The listing builds one solid part. Answer for the finished solid, in the listing's coordinates (mm). A direction names the side the tool comes from. Give positions to 0.01 mm unless a question says otherwise; leave off trailing zeros. Order: outer loops, then holes, each group sorted by start corner. A loop starts at its lowest first (then second) coordinate and runs counter-clockwise, first axis right, second up. Notation, with made-up numbers: (47.5, 82.5) -> (105.5, 82.5) arc R33 ccw to (105.5, 118.5) -> close; hole circle Ø2 at (63, -17.75). An arc over 180 degrees is marked (long way). Answer as a JSON object with one key per item and string values. Group by question number.
```python
from build123d import *

# Parameters (mm, degrees)
CYLINDER004_R     = 36.5
CYLINDER004_DEPTH = 4
CYLINDER005_R     = 38
CYLINDER005_DEPTH = 4
CYLINDER003_R     = 36.5
CYLINDER003_DEPTH = 4
CYLINDER002_R     = 38
CYLINDER002_DEPTH = 4
CYLINDER001_R     = 1.5
CYLINDER001_DEPTH = 40
CYLINDER_R        = 35
CYLINDER_DEPTH    = 35
PAD_DEPTH         = 1
SKETCH001_R       = 3
HOLE_DEPTH        = 25
PAD001_DEPTH      = 18
FILLET_1_R        = 1
FILLET_2_R        = 0.9
FILLET001_R       = 1
FILLET002_R       = 0.3


with BuildPart() as cylinder004:
    # Cylinder004 → Cylinder004 (new body)
    with BuildSketch(Plane(origin=(0, 0, -45), x_dir=(1, 0, 0), z_dir=(0, -1, 0))):
        Circle(CYLINDER004_R)
    extrude(amount=CYLINDER004_DEPTH)


with BuildPart() as cut003:
    # Cylinder005 → Cylinder005 (new body)
    with BuildSketch(Plane(origin=(0, 0, -45), x_dir=(1, 0, 0), z_dir=(0, -1, 0))):
        Circle(CYLINDER005_R)
    extrude(amount=CYLINDER005_DEPTH)

    # Cut003: cut Cylinder004
    add(cylinder004.part, mode=Mode.SUBTRACT)


with BuildPart() as cut003_1:
    # Cut003 placement: moved
    add(cut003.part.moved(Location((0, -12, 0))))


with BuildPart() as cylinder003:
    # Cylinder003 → Cylinder003 (new body)
    with BuildSketch(Plane(origin=(0, 0, -45), x_dir=(1, 0, 0), z_dir=(0, -1, 0))):
        Circle(CYLINDER003_R)
    extrude(amount=CYLINDER003_DEPTH)


with BuildPart() as fusion:
    # Cylinder002 → Cylinder002 (new body)
    with BuildSketch(Plane(origin=(0, 0, -45), x_dir=(1, 0, 0), z_dir=(0, -1, 0))):
        Circle(CYLINDER002_R)
    extrude(amount=CYLINDER002_DEPTH)

    # Cut002: cut Cylinder003
    add(cylinder003.part, mode=Mode.SUBTRACT)


with BuildPart() as fusion_1:
    # Cut002 placement: moved
    add(fusion.part.moved(Location((0, 6, 0))))

    # Fusion: union Cut003
    add(cut003_1.part)


with BuildPart() as cylinder001:
    # Cylinder001 → Cylinder001 (new body)
    with BuildSketch(Plane(origin=(-20, -15.75, -9.5), x_dir=(0, 0, -1), z_dir=(1, 0, 0))):
        Circle(CYLINDER001_R)
    extrude(amount=CYLINDER001_DEPTH)


with BuildPart() as cylinder:
    # Cylinder → Cylinder (new body)
    with BuildSketch(Plane(origin=(0, 12, -45), x_dir=(1, 0, 0), z_dir=(0, -1, 0))):
        Circle(CYLINDER_R)
    extrude(amount=CYLINDER_DEPTH)


with BuildPart() as fillet002:
    # Sketch → Pad (new body)
    with BuildSketch(Plane.XY):
        with BuildLine():
            ThreePointArc((-16, 10.5), (-18.474874, 9.474874), (-19.5, 7))
            Line((-19.5, 7), (-19.5, -17))
            ThreePointArc((-19.5, -17), (-18.474874, -19.474874), (-16, -20.5))
            Line((-16, -20.5), (15.999994, -20.5))
            ThreePointArc((15.999994, -20.5), (18.474872, -19.474876), (19.5, -17))
            Line((19.5, -17), (19.5, 7))
            ThreePointArc((19.5, 7), (18.474874, 9.474874), (16, 10.5))
            Line((16, 10.5), (-16, 10.5))
        make_face()
    extrude(amount=PAD_DEPTH)

    # Sketch001 (on Face9 of Pad) → Hole (cut)
    with BuildSketch(Plane(origin=(0, 0, 0), x_dir=(1, 0, 0), z_dir=(0, 0, -1))):
        Circle(SKETCH001_R)
    extrude(amount=-HOLE_DEPTH, mode=Mode.SUBTRACT)

    # Sketch002 (on Face4 of Hole) → Pad001 (join)
    with BuildSketch(Plane(origin=(0, 0, 0), x_dir=(1, 0, 0), z_dir=(0, 0, -1))):
        with BuildLine():
            Line((-16, 20.5), (15.999994, 20.5))
            ThreePointArc((19.5, 17), (18.474872, 19.474876), (15.999994, 20.5))
            Line((19.5, 17), (19.5, -7))
            ThreePointArc((16, -10.5), (18.474874, -9.474874), (19.5, -7))
            Line((16, -10.5), (-16, -10.5))
            ThreePointArc((-19.5, -7), (-18.474874, -9.474874), (-16, -10.5))
            Line((-19.5, -7), (-19.5, 17))
            ThreePointArc((-16, 20.5), (-18.474874, 19.474874), (-19.5, 17))
        make_face()
        with BuildLine():
            ThreePointArc((-18.5, -7), (-17.767767, -8.767767), (-16, -9.5))
            Line((16, -9.5), (-16, -9.5))
            ThreePointArc((16, -9.5), (17.767767, -8.767767), (18.5, -7))
            Line((18.5, 17), (18.5, -7))
            ThreePointArc((18.5, 17), (17.767767, 18.767767), (16, 19.5))
            Line((-15.993973, 19.5), (16, 19.5))
            ThreePointArc((-15.993973, 19.5), (-17.767772, 18.767772), (-18.5, 16.993973))
            Line((-18.5, -7), (-18.5, 16.993973))
        make_face(mode=Mode.SUBTRACT)
    extrude(amount=PAD001_DEPTH)

    # Cut: cut Cylinder
    add(cylinder.part, mode=Mode.SUBTRACT)

    # Cut001: cut Cylinder001
    add(cylinder001.part, mode=Mode.SUBTRACT)

    # Fillet 1
    fillet_1_edges = [fillet002.edges().sort_by_distance(p)[0] for p in [
        (0.003014, -19.5, 0),
    ]]
    fillet(fillet_1_edges, radius=FILLET_1_R)

    # Fillet 2
    fillet_2_edges = [fillet002.edges().sort_by_distance(p)[0] for p in [
        (19.5, -5, 1),
    ]]
    fillet(fillet_2_edges, radius=FILLET_2_R)

    # Cut004: cut Fusion
    add(fusion_1.part, mode=Mode.SUBTRACT)

    # Fillet001
    fillet001_edges = [fillet002.edges().sort_by_distance(p)[0] for p in [
        (-19.5, 4, -14.145503),
        (-19.5, -14, -14.145503),
        (19.5, -14, -14.145503),
        (19.5, 4, -14.145503),
    ]]
    fillet(fillet001_edges, radius=FILLET001_R)

    # Fillet002
    fillet002_edges = [fillet002.edges().sort_by_distance(p)[0] for p in [
        (-18.5, 4, -13.535735),
        (-18.5, -14, -13.535735),
        (18.5, -14, -13.535735),
        (18.5, 4, -13.535735),
    ]]
    fillet(fillet002_edges, radius=FILLET002_R)


solid = fillet002.part
```
(1) A cutting plane is placed at A-A (y = 3.5). Determine the outline of the cut face in (x, z), and give its area (3 significant figures).
(2) Flat-ended cylindrical pins translate along their axes: pin 1 Ø5 at (x, y) = (-2, -11) entering from -Z; pin 2 Ø0.5 at (x, z) = (19, -13.5) entering from -Y; pin 3 Ø0.5 at (x, z) = (19, -13.5) entering from +Y. Find the tip coordinate at first contact, or state that the pin passes through.
(3) A cutting plane is placed at C-C (y = 0). Determine the outline of the cut face in (x, z).
(4) A cutting plane is placed at D-D (z = -9.5). Determine the outline of the cut face in (x, y).
(5) Which of the six approach directions +Z, -Z, +X, -X, +Y, -Y give full straight-line access (tool end or side, diameter ignored) to faces 5 (the cylindrical face through (18.215, -4.832, -0.301)), 6 (the cylindrical face through (19.009, 4.028, -12.096)), 7 (the cylindrical face through (19, -15.7, -8))?
(6) For a pull along Z with two mould halves and no side action, classify faces 1 (the cylindrical face through (-0.22, 10.24, 0.73)), 2 (the cylindrical face through (-3, -0.1, 0.5)), 3 (the cylindrical face through (-19.376, 4.028, -14.218)), 4 (the cylindrical face through (0.227, -19.215, -0.301)) as +Z half, -Z half, draft (parallel to the pull), parting line (faces both ways), or undercut.
(7) Find the intervals of material crossed by line 1 along X through (y, z) = (3.5, -5.25); line 2 along Y through (x, z) = (14, -9); line 3 along Z through (x, y) = (14, 8), in increasing order. Write a range as [from, to].
(8) A cutting plane is placed at B-B (x = 0). Determine the outline of the cut face in (y, z), and give its area (3 significant figures).
Check sheet entries:
{
 "1": {"outline": "(-19.5, -15.94) arc R35 cw to (-18.5, -15.29) -> (-18.5, -14.06) arc R0.3 ccw to (-18.96, -13.81) arc R36.5 ccw to (-19.02, -13.85) arc R1 ccw to (-19.5, -14.7) -> close; (-19.5, -12.38) arc R38 cw to (-18.5, -11.81) -> (-18.5, -1) arc R1 cw to (-17.5, 0) -> (17.5, 0) arc R1 cw to (18.5, -1) -> (18.5, -11.81) arc R38 cw to (19.5, -12.38) -> (19.5, 0.1) arc R0.9 ccw to (18.6, 1) -> (-18.6, 1) arc R0.9 ccw to (-19.5, 0.1) -> close; (18.5, -15.29) arc R35 cw to (19.5, -15.94) -> (19.5, -14.7) arc R1 ccw to (19.02, -13.85) arc R36.5 ccw to (18.96, -13.81) arc R0.3 ccw to (18.5, -14.06) -> close", "area": "66.6 mm2"},
 "2": {"pin 1": "stops at z = 0", "pin 2": "stops at y = -19.17", "pin 3": "stops at y = 9.17"},
 "3": {"outline": "(-19.5, -15.94) arc R35 cw to (-18.5, -15.29) -> (-18.5, -1) arc R1 cw to (-17.5, 0) -> (-3, 0) -> (-3, 1) -> (-18.6, 1) arc R0.9 ccw to (-19.5, 0.1) -> close; (3, 0) -> (17.5, 0) arc R1 cw to (18.5, -1) -> (18.5, -15.29) arc R35 cw to (19.5, -15.94) -> (19.5, 0.1) arc R0.9 ccw to (18.6, 1) -> (3, 1) -> close"},
 "4": {"outline": "(-19.5, -14.25) -> (-18.5, -14.25) -> (-18.5, 7) arc R2.5 cw to (-16, 9.5) -> (16, 9.5) arc R2.5 cw to (18.5, 7) -> (18.5, -14.25) -> (19.5, -14.25) -> (19.5, 7) arc R3.5 ccw to (16, 10.5) -> (-16, 10.5) arc R3.5 ccw to (-19.5, 7) -> close; (-19.49, -17.25) arc R3.5 ccw to (-16, -20.5) -> (16, -20.5) arc R3.5 ccw to (19.49, -17.25) -> (18.49, -17.25) arc R2.5 cw to (16, -19.5) -> (-15.99, -19.5) arc R2.5 cw to (-18.49, -17.25) -> close"},
 "5": {"face 5": "-Z", "face 6": "none", "face 7": "+X, -X"},
 "6": {"face 1": "+Z half", "face 2": "draft", "face 3": "undercut", "face 4": "-Z half"},
 "7": {"line 1": "x = [-19.5, -18.5], [18.5, 19.5]", "line 2": "y = [-20.5, -19.5], [9.5, 10.5]", "line 3": "z = [0, 1]"},
 "8": {"outline": "(-20.5, -10) -> (-19.5, -10) -> (-19.5, -1) arc R1 cw to (-18.5, 0) -> (-3, 0) -> (-3, 1) -> (-19.6, 1) arc R0.9 ccw to (-20.5, 0.1) -> close; (3, 0) -> (8.5, 0) arc R1 cw to (9.5, -1) -> (9.5, -10) -> (10.5, -10) -> (10.5, 0.1) arc R0.9 ccw to (9.6, 1) -> (3, 1) -> close", "area": "45.1 mm2"}
}
